Autodesk Inventor part; units mm, degrees
ref_plane "ff_1_XY" through (0, 0, 0) normal (1, 0, 0) x (0, 0, -1)
ref_plane "ff_1_YZ" through (0, 0, 0) normal (0, 0, -1) x (0, 1, 0)
ref_plane "ff_1_ZX" through (0, 0, 0) normal (0, 1, 0) x (1, 0, 0)
sketch "Sketch_1" plane through (0, 0, 0) normal (0, 0, 1) x (1, 0, 0)
  line L0 (50, 0) -> (-50, 0)
  line L1 (-5, 11.5) -> (-4.5, 11)
  line L2 (-4.5, 11) -> (6.5, 11)
  line L3 (6.5, 11) -> (7, 11.5)
  line L4 (7, 11.5) -> (7, 21)
  line L5 (7, 21) -> (6.5, 21.5)
  line L6 (6.5, 21.5) -> (0.5, 21.5)
  line L7 (0.5, 21.5) -> (0, 21)
  line L8 (0, 21) -> (0, 14.25)
  arc A0 (-0.25, 14) -> (0, 14.25) centre (-0.25, 14.25) ccw
  line L9 (-0.25, 14) -> (-4.5, 14)
  line L10 (-4.5, 14) -> (-5, 13.5)
  line L11 (-5, 13.5) -> (-5, 11.5)
revolve "Revolution1" add sketch "Sketch_1" angle 360 about axis through (50, 0, 0) along (1, 0, 0)
sketch "Sketch_2" plane through (7, 0, 0) normal (1, 0, 0) x (0, 0, -1)
  line L0 (-49.4975, 0) -> (0, -49.4975)
  line L1 (0, -49.4975) -> (49.4975, 0)
  line L2 (49.4975, 0) -> (0, 49.4975)
  line L3 (0, 49.4975) -> (-49.4975, 0)
  line L4 (-24.7487, 0) -> (0, -24.7487)
  line L5 (0, -24.7487) -> (24.7487, 0)
  line L6 (24.7487, 0) -> (0, 24.7487)
  line L7 (0, 24.7487) -> (-24.7487, 0)
extrude "Extrusion1" cut sketch "Sketch_2" against normal blind 7
sketch "Sketch3" plane through (7, 0, 0) normal (1, 0, 0) x (0, 0, -1)
  point P0 (0, 17.5)
hole "Hole1" at (7, 17.5, 0) direction (-1, 0, 0) diameter 3.4 depth 7 counterbore diameter 6.5 counterbore depth 4
pattern_linear "Rectangular Pattern1" count 2 spacing 24.7487 along (0, -0.7071, 0.7071) count 2 spacing 24.7487 along (0, -0.7071, -0.7071) of "Hole1"
ref_plane "ff_1_XY" through (0, 0, 0) normal (1, 0, 0) x (0, 0, -1)
ref_plane "ff_1_YZ" through (0, 0, 0) normal (0, 0, -1) x (0, 1, 0)
ref_plane "ff_1_ZX" through (0, 0, 0) normal (0, 1, 0) x (1, 0, 0)
ref_plane "ff_2x_XY" through (1, 0, 0) normal (1, 0, 0) x (0, 0, -1)
ref_plane "ff_2x_YZ" through (1, 0, 0) normal (0, 0, -1) x (0, 1, 0)
ref_plane "ff_2x_ZX" through (1, 0, 0) normal (0, 1, 0) x (1, 0, 0)
properties part number "FF 10Part1"
Model file for the job. Use its own axes, mm. A direction names the side the tool comes from. Coordinates: 2 decimals unless noted, no trailing zeros. Order: outer loops, then holes, each group sorted by start corner. A loop starts at its lowest first (then second) coordinate and runs counter-clockwise, first axis right, second up. Notation, with made-up numbers: (39, 3.25) -> (88, 3.25) arc R34 cw to (88, 34.25) -> close; hole circle Ø10 at (-36, 3). An arc over 180 degrees is marked (long way). Answer as a JSON object with one key per item and string values. Group by question number.
1) Cut at B-B, the plane x = 2. Write the cut outline in (y, z), then the cut area to 3 significant figures.
2) Flat gauge pins, fed straight in: pin 1 (6 mm diameter, centred on y = 0, z = 17.5, fed in from +X); pin 2 (3 mm diameter, centred on x = 3.5, z = 16.5, fed in from +Y); pin 3 (5 mm diameter, centred on y = -1.5, z = -8, fed in from +X); pin 4 (4 mm diameter, centred on y = 9, z = -1.5, fed in from +X). Where does each tip first touch, or does it go through?
3) Cut at C-C, the plane y = -18. Write the cut outline in (x, z).
4) Cut at D-D, the plane z = 0. Count the separate pieces of the cut face and the enclosed holes in it, then the cut area to 3 significant figures.
5) Which spindle directions (+Z, -Z, +X, -X, +Y, -Y) get a long thin tool onto all of the face, cutting with end or side? Do faces 1 (the face through (4.972, -20.722, 0.423)), 2 (the face through (-2.405, 12.932, 5.362)), 3 (the face through (1.08, -2.38, -10.74)). Say none if no direction does.
6) Cut at A-A, the plane z = -17. Write the cut outline in (x, y), then the cut area to 3 significant figures.
7) Drill centre lines: L1, parallel to Y at x = 6, z = -18; L2, parallel to Y at x = 0.25, z = 16; L3, parallel to Z at x = 5.75, y = 17. Where is each one in solid material? Low to high.
8) Pull direction Z, two halves, no side cores. Call faces 4 (the face through (3.5, 21.5, 0)), 5 (the face through (1.479, 15.814, 0.221)), 6 (the face through (3.55, -12.5, -12.25)): +Z half, -Z half, draft (parallel to the pull), parting line (faces both ways), or undercut.
Check values:
{
 "1": {"outline": "(-21.21, -3.54) -> (-3.54, -21.21) arc R21.5 ccw to (3.54, -21.21) -> (21.21, -3.54) arc R21.5 ccw to (21.21, 3.54) -> (3.54, 21.21) arc R21.5 ccw to (-3.54, 21.21) -> (-21.21, 3.54) arc R21.5 ccw to start; hole circle Ø3.4 at (-17.5, 0); hole circle Ø22 at (0, 0); hole circle Ø3.4 at (0, -17.5); hole circle Ø3.4 at (0, 17.5); hole circle Ø3.4 at (17.5, 0)", "area": "764 mm²"},
 "2": {"pin 1": "stops at x = 3", "pin 2": "stops at y = 9.75", "pin 3": "passes through", "pin 4": "stops at x = 6.62"},
 "3": {"outline": "(0, -6.75) -> (7, -6.75) -> (7, -3.21) -> (3, -3.21) -> (3, -1.62) -> (0, -1.62) -> close; (0, 1.62) -> (3, 1.62) -> (3, 3.21) -> (7, 3.21) -> (7, 6.75) -> (0, 6.75) -> close"},
 "4": {"separate pieces": "4", "enclosed holes": "0", "area": "103 mm²"},
 "5": {"face 1": "+X", "face 2": "-X", "face 3": "+X, -X"},
 "6": {"outline": "(0, -7.75) -> (7, -7.75) -> (7, -3.21) -> (3, -3.21) -> (3, -1.62) -> (0, -1.62) -> close; (0, 1.62) -> (3, 1.62) -> (3, 3.21) -> (7, 3.21) -> (7, 7.75) -> (0, 7.75) -> close", "area": "73.0 mm²"},
 "7": {"L1": "y = -6.75 to -3.21, 3.21 to 6.75", "L2": "y = -8.75 to -0.8, 0.8 to 8.75", "L3": "z = -7.75 to -3.21, 3.21 to 7.75"},
 "8": {"face 4": "parting line", "face 5": "undercut", "face 6": "-Z half"}
}
